Model file for the job. Use its own axes, mm. Face numbers are marked on the shaded views. A direction names the side the tool comes from. Give positions to 0.01 mm unless a question says otherwise; leave off trailing zeros. Loops run counter-clockwise (first coordinate to the right, second up) from the corner with the lowest first, then second, coordinate; pieces in that order, holes last. Notation, with made-up numbers: M 78.5,83.5 L 128.5,83.5 A18 ccw 128.5,96.5 Z; hole C 48,72 d9. An arc over 180 degrees is marked long. Answer in a Markdown table with one row per item.
```python
from build123d import *

# Parameters (mm, degrees)
F0_R     = 20.955
F1_DEPTH = 2.54
F2_SIZE  = 1.905
F3_W     = 3.048
F3_H     = 16.51
F4_DEPTH = 4.572
F5_R     = 1.27
F6_R     = 0.381
F7_DEPTH = 25.4


with BuildPart() as f1:
    # F0 (on Top) → F1 (new body)
    with BuildSketch(Plane.XY):
        Circle(F0_R)
    extrude(amount=F1_DEPTH)

    # F2
    f2_edges = [f1.edges().sort_by_distance(p)[0] for p in [
        (-20.955, 0, 2.54),
    ]]
    chamfer(f2_edges, length=F2_SIZE)

    # F3 (on Top) → F4 (join)
    with BuildSketch(Plane.XY):
        with Locations((-19.812, 0)):
            Rectangle(F3_W, F3_H)
    extrude(amount=F4_DEPTH)

    # F5
    f5_edges = [f1.edges().sort_by_distance(p)[0] for p in [
        (-21.336, 0, 4.572),
    ]]
    fillet(f5_edges, radius=F5_R)

    # F6 (on face) → F7 (cut)
    with BuildSketch(Plane.XZ.offset(8.255)):
        with Locations((-20.066, 3.302)):
            Circle(F6_R)
    extrude(amount=-F7_DEPTH, mode=Mode.SUBTRACT)


solid = f1.part
```
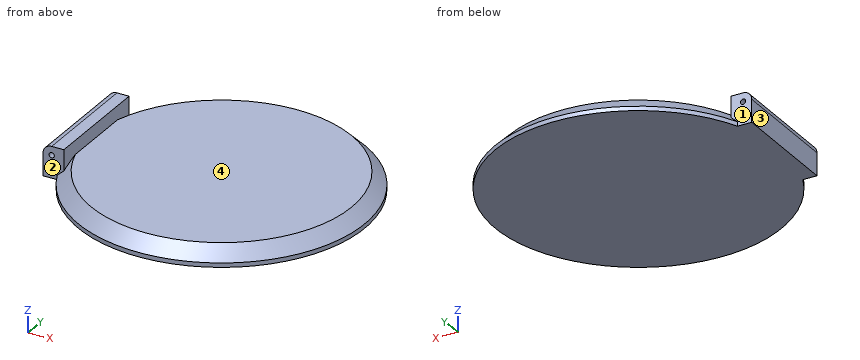
(1) Saw through at B-B, the plane x = 0. Give the cut face in (y, z) (3 decimals), and give its area (3 significant figures).
Established:
| item | result |
|---|---|
| outline | M -20.955,0 L 20.955,0 L 20.955,0.635 L 19.05,2.54 L -19.05,2.54 L -20.955,0.635 Z |
| area | 103 mm2 |
(2) Which spindle directions (+Z, -Z, +X, -X, +Y, -Y) get a long thin tool onto all of the face, cutting with end or side? Do the marked faces 1, 2, 3 and 4. Say none if no direction does.
Established:
| item | result |
|---|---|
| face 1 | +Z, -X, +Y |
| face 2 | +Z, -X, -Y |
| face 3 | +Z, -Z, -X, +Y, -Y |
| face 4 | +Z, +X, +Y, -Y |
(3) Wall check: L1, parallel to Z at x = -17, y = -5; L2, parallel to X at y = -2.5, z = 3.6; L3, parallel to X at y = -8, z = 1.45. Give the ranges that are in metal, low to high.
Established:
| item | result |
|---|---|
| L1 | z = 0 to 2.54 |
| L2 | x = -21.3 to -20.3, -19.83 to -18.29 |
| L3 | x = -21.34 to 18.48 |
(4) Flat gauge pins, fed straight in: P1, Ø0.9, axis at x = -20, z = 2.5, coming from the -Y side (3 decimals); P2, Ø4, axis at x = 10.5, y = -2, coming from the +Z side; P3, Ø2.5, axis at x = -19.5, z = 3, coming from the +Y side (3 decimals). Where does each tip first touch, or does it go through?
Established:
| item | result |
|---|---|
| P1 | stops at y = -8.255 |
| P2 | stops at z = 2.54 |
| P3 | stops at y = 8.255 |
(5) Saw through at A-A, the plane y = 0. Give the cut face in (x, z) (3 decimals).
Established:
| item | result |
|---|---|
| outline | M -21.336,0 L 20.955,0 L 20.955,0.635 L 19.05,2.54 L -18.288,2.54 L -18.288,4.572 L -20.066,4.572 A1.27 ccw -21.336,3.302 Z; hole C -20.066,3.302 d0.762 |
